For this review, take the finished solid that the model builds, in its own axes (mm). Round coordinates to 2 decimals unless told otherwise and drop trailing zeros. Write each loop counter-clockwise with the first axis right and the second up, starting at its lowest first coordinate (ties: lowest second). Pieces come first, ordered by that corner, then holes. Notation, with made-up numbers: M 4.25,8 L 46.25,8 A20 ccw 46.25,33 Z; hole C 57.5,-28 d8. An arc over 180 degrees is marked long. Answer in a Markdown table with one row per item.
```python
from build123d import *

# Parameters (mm, degrees)
F0_W     = 25.4
F0_H     = 25.4
F0_W_2   = 2235.2
F0_H_2   = 558.8
F1_DEPTH = 25.4
F2_DEPTH = 152.4
F4_W     = 2286
F4_H     = 609.6
F4_W_2   = 2235.2
F4_H_2   = 558.8
F5_DEPTH = 25.4


with BuildPart() as f1:
    # F0 (on Top) → F1 (new body)
    with BuildSketch(Plane.XY):
        with Locations((-1130.3, -292.1)):
            Rectangle(F0_W, F0_H)
        with Locations((0, -292.1)):
            Rectangle(F0_W_2, F0_H)
        with Locations((-1130.3, 0)):
            Rectangle(F0_W, F0_H_2)
        with Locations((1130.3, -292.1)):
            Rectangle(F0_W, F0_H)
        with Locations((-1130.3, 292.1)):
            Rectangle(F0_W, F0_H)
        with Locations((1130.3, 0)):
            Rectangle(F0_W, F0_H_2)
        with Locations((0, 292.1)):
            Rectangle(F0_W_2, F0_H)
        with Locations((1130.3, 292.1)):
            Rectangle(F0_W, F0_H)
    extrude(amount=-F1_DEPTH)

    # F0 (on Top) → F2 (join)
    with BuildSketch(Plane.XY):
        with Locations((-1130.3, 292.1)):
            Rectangle(F0_W, F0_H)
        with Locations((-1130.3, -292.1)):
            Rectangle(F0_W, F0_H)
        with Locations((1130.3, 292.1)):
            Rectangle(F0_W, F0_H)
        with Locations((1130.3, -292.1)):
            Rectangle(F0_W, F0_H)
    extrude(amount=F2_DEPTH)

    # F4 (on offset) → F5 (join)
    with BuildSketch(Plane.XY.offset(152.4)):
        Rectangle(F4_W, F4_H)
        Rectangle(F4_W_2, F4_H_2, mode=Mode.SUBTRACT)
    extrude(amount=-F5_DEPTH)


solid = f1.part
```
Q1. Take a section at A-A (z = 79). State the section outline as (x, y) points.
Found:
| item | result |
|---|---|
| outline | M -1143,-304.8 L -1117.6,-304.8 L -1117.6,-279.4 L -1143,-279.4 Z; M -1143,279.4 L -1117.6,279.4 L -1117.6,304.8 L -1143,304.8 Z; M 1117.6,-304.8 L 1143,-304.8 L 1143,-279.4 L 1117.6,-279.4 Z; M 1117.6,279.4 L 1143,279.4 L 1143,304.8 L 1117.6,304.8 Z |
Q2. For probe 1 along X at (y, z) = (22.5, -4); probe 2 along Y at (x, z) = (744, -3.5), list the stretches that pass through material, from the lowest coordinate up.
Found:
| item | result |
|---|---|
| probe 1 | -1143 to -1117.6, 1117.6 to 1143 |
| probe 2 | -304.8 to -279.4, 279.4 to 304.8 |
Q3. Take a section at B-B (y = -97). State the section outline as (x, z) points.
Found:
| item | result |
|---|---|
| outline | M -1143,-25.4 L -1117.6,-25.4 L -1117.6,0 L -1143,0 Z; M -1143,127 L -1117.6,127 L -1117.6,152.4 L -1143,152.4 Z; M 1117.6,-25.4 L 1143,-25.4 L 1143,0 L 1117.6,0 Z; M 1117.6,127 L 1143,127 L 1143,152.4 L 1117.6,152.4 Z |
Q4. Insertion check: P1, Ø8, axis at y = 175, z = 120, coming from the +X side. The pin has a flat end and moves straight along its axis. Give the tip position at first contact, or say it passes through.
Found:
| item | result |
|---|---|
| P1 | through |
